```python
from build123d import *

# Parameters (mm, degrees)
BOSS_EXTRUDE1_DEPTH          = 2.54
FILLET1_R                    = 2.54
F_39_0_0995_DIAMETER_HOLE1_D = 2.5273


with BuildPart() as part:
    # Sketch1 → Boss-Extrude1 (new body)
    with BuildSketch(Plane.XY):
        Polygon((0, 0), (0, 76.2), (5.08, 76.2), (5.08, 30.48), (30.48, 30.48), (30.48, 76.2), (35.56, 76.2), (35.56, 0), align=None)
    extrude(amount=BOSS_EXTRUDE1_DEPTH)

    # Fillet1
    fillet1_edges = [part.edges().sort_by_distance(p)[0] for p in [
        (5.08, 30.48, 1.27),
        (30.48, 30.48, 1.27),
    ]]
    fillet(fillet1_edges, radius=FILLET1_R)

    # #39 (0.0995) Diameter Hole1 (through all)
    with Locations(Plane.XY.offset(2.54)):
        with Locations((32.820840104, 68.709866644), (32.784904498, 51.685945396), (32.816003505, 34.693675088), (26.329237865, 28.403700876), (9.329223304, 28.403700876), (2.784904498, 34.68594536), (2.816003505, 51.696905496), (2.816003505, 68.709866644)):
            Hole(F_39_0_0995_DIAMETER_HOLE1_D / 2)


solid = part.part
```
The listing builds one solid part. Answer for the finished solid, in the listing's coordinates (mm). A direction names the side the tool comes from. Coordinates: 2 decimals unless noted, no trailing zeros. Loops run counter-clockwise (first coordinate to the right, second up) from the corner with the lowest first, then second, coordinate; pieces in that order, holes last. Notation, with made-up numbers: (44, 55) - (94, 55) arc R10 cw to (94, 74) - close; hole circle Ø8 at (25, -33.75). An arc over 180 degrees is marked (long way). Write item = value, one per line.
1) Section B-B (x = 16) is taken. Determine the outline of the cut face in (y, z).
Responses:
outline = (0, 0) - (30.48, 0) - (30.48, 2.54) - (0, 2.54) - close
2) Determine the mould class of faces 1 (the face through (9.6, 27.17, 1.25)), 2 (the face through (32.14, 35.76, 1.25)), 3 (the face through (18, 30.48, 1)), 4 (the face through (5.08, 55, 1)) for opening direction Y: pulls with the +Y half, pulls with the -Y half, needs draft (parallel to the pull), parting line crosses it, or undercut.
Responses:
face_1 = undercut
face_2 = undercut
face_3 = pulls with the +Y half
face_4 = needs draft
3) Which of the six approach directions +Z, -Z, +X, -X, +Y, -Y give full straight-line access (tool end or side, diameter ignored) to faces 5 (the face through (30.48, 54, 1)), 6 (the face through (18, 22, 0))?
Responses:
face_5 = +Z, -Z, +Y
face_6 = -Z, +X, -X, +Y, -Y
4) Find the intervals of material crossed by line 1 along X through (y, z) = (28.5, 0.75); line 2 along X through (y, z) = (55, 1); line 3 along X through (y, z) = (28, 1.55), in increasing order.
Responses:
line_1 = 0 to 8.07, 10.59 to 25.07, 27.59 to 35.56
line_2 = 0 to 5.08, 30.48 to 35.56
line_3 = 0 to 8.13, 10.53 to 25.13, 27.53 to 35.56
5) Section A-A (y = 60) is taken. Determine the outline of the cut face in (x, z).
Responses:
outline = (0, 0) - (5.08, 0) - (5.08, 2.54) - (0, 2.54) - close; (30.48, 0) - (35.56, 0) - (35.56, 2.54) - (30.48, 2.54) - close
6) Section C-C (z = 0.6) is taken. Count the separate pieces of the cut face and the enclosed holes in it, plus the area to 3 significant figures.
Responses:
separate_pieces = 1
enclosed_holes = 8
area = 1,510 mm^2
